For this review, take the finished solid that the model builds, in its own axes (mm). Face numbers are marked on the shaded views. Round coordinates to 2 decimals unless told otherwise and drop trailing zeros. Order: outer loops, then holes, each group sorted by start corner. A loop starts at its lowest first (then second) coordinate and runs counter-clockwise, first axis right, second up. Notation, with made-up numbers: (-1.5, -39.75) - (47.5, -39.75) arc R16 cw to (47.5, -28.75) - close; hole circle Ø11 at (-33, -21). An arc over 180 degrees is marked (long way). One line per item, written item: value.
```python
from build123d import *

# Parameters (mm, degrees)
SKETCH2_R             = 15
SKETCH2_R_2           = 12.5
BOSS_EXTRUDE1_DEPTH   = 10
SKETCH2_R_3           = 7.5
SKETCH2_R_4           = 5
BOSS_EXTRUDE1_2_DEPTH = 10
SKETCH2_3_R           = 12.5
SKETCH2_3_R_2         = 7.5
BOSS_EXTRUDE2_DEPTH   = 9


with BuildPart() as part:
    # Sketch2 → Boss-Extrude1 (new body)
    with BuildSketch(Plane.XY):
        Circle(SKETCH2_R)
        Circle(SKETCH2_R_2, mode=Mode.SUBTRACT)
    extrude(amount=BOSS_EXTRUDE1_DEPTH)



with BuildPart() as body_2:
    # Sketch2 → Boss-Extrude1 2 (new body)
    with BuildSketch(Plane.XY):
        Circle(SKETCH2_R_3)
        Circle(SKETCH2_R_4, mode=Mode.SUBTRACT)
    extrude(amount=BOSS_EXTRUDE1_2_DEPTH)


with BuildPart() as part_1:
    add(part.part)

    add(body_2.part)  # Boss-Extrude2 merges body 2
    # Sketch2_3 → Boss-Extrude2 (add)
    with BuildSketch(Plane.XY):
        Circle(SKETCH2_3_R)
        Circle(SKETCH2_3_R_2, mode=Mode.SUBTRACT)
    extrude(amount=BOSS_EXTRUDE2_DEPTH)


solid = part_1.part
```
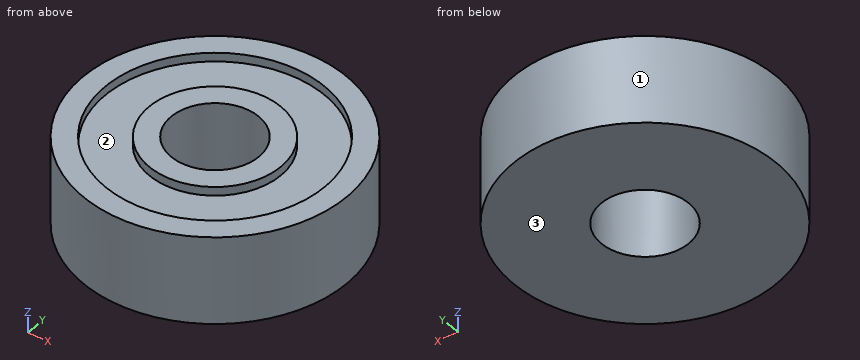
Item 1: Wall thickness on line 1 (Y direction, x = 0, z = 9.7); line 2 (Y direction, x = 0, z = 6.5); line 3 (X direction, y = 1.5, z = 5): over which ranges is each line inside the solid? List them lowest first.
Returned:
line 1: -15 to -12.5, -7.5 to -5, 5 to 7.5, 12.5 to 15
line 2: -15 to -5, 5 to 15
line 3: -14.92 to -4.77, 4.77 to 14.92
Item 2: Take a section at D-D (z = 8.5). Write out the cut boundary in (x, y), plus the area to 3 significant figures.
Returned:
outline: circle Ø30 at (0, 0); hole circle Ø10 at (0, 0)
area: 628 mm^2
Item 3: Take a section at C-C (x = 12). Write out the cut boundary in (y, z), plus the area to 3 significant figures.
Returned:
outline: (-9, 0) - (9, 0) - (9, 10) - (3.5, 10) - (3.5, 9) - (-3.5, 9) - (-3.5, 10) - (-9, 10) - close
area: 173 mm^2
Item 4: Take a section at A-A (y = 0). Write out the cut boundary in (x, z).
Returned:
outline: (-15, 0) - (-5, 0) - (-5, 10) - (-7.5, 10) - (-7.5, 9) - (-12.5, 9) - (-12.5, 10) - (-15, 10) - close; (5, 0) - (15, 0) - (15, 10) - (12.5, 10) - (12.5, 9) - (7.5, 9) - (7.5, 10) - (5, 10) - close
Item 5: For P1, Ø6, axis at x = 7.5, z = 4, coming from the +Y side; P2, Ø1, axis at y = 9.5, z = 1.5, coming from the -X side, all flat-tipped, find the tip position at first contact; note any pin that passes through.
Returned:
P1: y = 14.31
P2: x = -12
Item 6: The part is to be moulded in two halves that separate along Y. For the marked faces 1, 2 and 3, say which applies: +Y half, -Y half, draft (parallel to the pull), parting line (faces both ways), or undercut.
Returned:
face 1: parting line
face 2: undercut
face 3: draft
